from build123d import *

# Parameters (mm, degrees)
F0_W     = 5
F0_H     = 10
F1_DEPTH = 1.4
F2_T     = -0.9
F4_DEPTH = 0.8


with BuildPart() as f1:
    # F0 (on Top) → F1 (new body)
    with BuildSketch(Plane.XY):
        with Locations((3.4046815708, 2.8265781289)):
            Rectangle(F0_W, F0_H)
    extrude(amount=F1_DEPTH)

    # F2
    f2_openings = [f1.faces().sort_by_distance(p)[0] for p in [
        (3.404682, 2.826578, 1.4),
    ]]
    offset(amount=F2_T, openings=f2_openings)

    # F3 (on face) → F4 (join)
    with BuildSketch(Plane.XY.offset(0.9)):
        Polygon((5.0046815708, -0.2734218711), (5.0046815708, 0.6265781289), (3.4046815708, 0.6265781289), (3.4046815708, 2.1265781289), (4.3046815708, 2.1265781289), (4.3046815708, 5.9265781289), (2.5046815708, 5.9265781289), (2.5046815708, -0.2734218711), align=None)
    extrude(amount=F4_DEPTH)


solid = f1.part
Design review of the part built by this model. Coordinates are the model's own, in mm. A direction names the side the tool comes from. Give positions to 0.01 mm unless a question says otherwise; leave off trailing zeros. Loops run counter-clockwise (first coordinate to the right, second up) from the corner with the lowest first, then second, coordinate; pieces in that order, holes last. Notation, with made-up numbers: M 59.5,-35.75 L 64.5,-35.75 A25 ccw 64.5,1.25 Z; hole C -15,80 d8. An arc over 180 degrees is marked long. One line per question, with ' | ' between items. Start each with the question number.
1. The part is to be moulded in two halves that separate along X. For faces 1 (the face through (5.905, 3, 1)), 2 (the face through (3.74, 1.97, 0.9)), 3 (the face through (3, 7.827, 1)), say which applies: released by +X, released by -X, zero draft, split by the parting line, or undercut.
2. Add section C-C (y = 1). Write out the cut boundary in (x, z).
3. Add section B-B (x = 3.6). Write out the cut boundary in (y, z).
4. To check wall thickness, follow L1, parallel to X at y = 2, z = 1.3; L2, parallel to X at y = 5.5, z = 1.35; L3, parallel to Y at x = 4.15, z = 0.95. State the ranges of each line that lie inside material, in increasing order.
5. Add section D-D (z = 1.55). Write out the cut boundary in (x, y).
6. For faces 4 (the face through (4.305, 4, 1.3)), 5 (the face through (0.905, 3, 1)), list the 3-axis set-ups (+Z, -Z, +X, -X, +Y, -Y) from which the entire face can be reached by the end or side of a thin tool; tool diameter is ignored.
7. Add section A-A (z = 1.05). Write out the cut boundary in (x, y), plus the area to 3 significant figures.
Worked out:
1) face 1: released by +X | face 2: undercut | face 3: zero draft
2) outline: M 0.9,0 L 5.9,0 L 5.9,1.4 L 5,1.4 L 5,0.9 L 3.4,0.9 L 3.4,1.7 L 2.5,1.7 L 2.5,0.9 L 1.8,0.9 L 1.8,1.4 L 0.9,1.4 Z
3) outline: M -2.17,0 L 7.83,0 L 7.83,1.4 L 6.93,1.4 L 6.93,0.9 L 5.93,0.9 L 5.93,1.7 L 2.13,1.7 L 2.13,0.9 L 0.63,0.9 L 0.63,1.7 L -0.27,1.7 L -0.27,0.9 L -1.27,0.9 L -1.27,1.4 L -2.17,1.4 Z
4) L1: x = 0.9 to 1.8, 2.5 to 3.4, 5 to 5.9 | L2: x = 0.9 to 1.8, 2.5 to 4.3, 5 to 5.9 | L3: y = -2.17 to -1.27, -0.27 to 0.63, 2.13 to 5.93, 6.93 to 7.83
5) outline: M 2.5,-0.27 L 5,-0.27 L 5,0.63 L 3.4,0.63 L 3.4,2.13 L 4.3,2.13 L 4.3,5.93 L 2.5,5.93 Z
6) face 4: +Z | face 5: +Z, -Z, -X, +Y, -Y
7) outline: M 0.9,-2.17 L 5.9,-2.17 L 5.9,7.83 L 0.9,7.83 Z; hole M 1.8,-1.27 L 5,-1.27 L 5,-0.27 L 2.5,-0.27 L 2.5,5.93 L 4.3,5.93 L 4.3,2.13 L 3.4,2.13 L 3.4,0.63 L 5,0.63 L 5,6.93 L 1.8,6.93 Z | area: 34.2 mm²
